Check sheet for the modelled part. Datum: model origin and axes. Units: mm. Coordinates: 2 decimals unless noted, no trailing zeros. Loops run counter-clockwise (first coordinate to the right, second up) from the corner with the lowest first, then second, coordinate; pieces in that order, holes last. Notation, with made-up numbers: M 20,84 L 77,84 A17 cw 77,93 Z; hole C 19,-40 d10. An arc over 180 degrees is marked long. Use CSV: the item, a comma, the result in double quotes. Start each with the question number.
(1) Scan lines: line 1 (Z direction, x = 9, y = 4.25); line 2 (Z direction, x = -8.5, y = 5.25); line 3 (Z direction, x = -76.5, y = 9.25). Record each from-to range of solid material in increasing order.
(2) Go/stop test with flat-tipped pins: pin 1 Ø6.5 at (y, z) = (4.5, -38) entering from -X; pin 2 Ø12 at (x, z) = (12.5, 74.5) entering from +Y; pin 3 Ø2 at (y, z) = (6, -51.5) entering from -X. Record where each tip stops, or that it passes through.
(3) Section check B-B on x = -17. Record the cut outline in (y, z), and give its area (3 significant figures).
(4) Section check C-C on z = 66. Record the cut outline in (x, y).
(5) Section check D-D on y = 2.5. Give the number of separate pieces and of enclosed holes in the cut face, and give its area (3 significant figures).
(6) Draft check along X on faces 1 (the flat face through (-74, 10, 62)), 2 (the flat face through (-89.5, 5, -39)), 3 (the cylindrical face through (-3.905, 6.338, -0.867)), 4 (the flat face through (89.5, 5, -47)). Enter one of: pulls with the +X half, pulls with the -X half, needs draft (parallel to the pull), parting line crosses it, or undercut.
(7) Section check A-A on x = -42.5. Record the cut outline in (y, z).
from build123d import *

# Parameters (mm, degrees)
SKETCH1_W               = 32.5
SKETCH1_H               = 40
SKETCH1_R               = 1.55
SKETCH1_W_2             = 40
SKETCH1_H_2             = 32.75
BOSS_EXTRUDE1_DEPTH     = 10
BOSS_EXTRUDE2_DEPTH     = 12.5
SKETCH3_R               = 4
CUT_EXTRUDE1_DEPTH      = 12.5
FILL_PATTERN1_OUTLINE_R = 4
FILL_PATTERN1_DEPTH     = 12.5
FILLET1_R               = 10
FILLET2_R               = 2


# Read off the part's stored shape, not the designer's step: Fill Pattern1
with BuildPart() as part:
    # Sketch1 → Boss-Extrude1 (new body)
    # profile 1 of 9: a face of its own
    with BuildSketch(Plane(origin=(0, 0, 0), x_dir=(1, 0, 0), z_dir=(0, 1, 0))):
        with BuildLine():
            Line((-35, 62.25), (-72, 62.25))
            ThreePointArc((-72, 62.25), (-77.125631329, 49.875631329), (-89.5, 44.75))
            Line((-89.5, 44.75), (-89.5, 35))
            Line((-89.5, 35), (-86.5, 35))
            Line((-86.5, 35), (-86.5, 20))
            Line((-86.5, 20), (-57, 20))
            Line((-57, 20), (-57, -20))
            Line((-57, -20), (-86.5, -20))
            Line((-86.5, -20), (-86.5, -35))
            Line((-86.5, -35), (-89.5, -35))
            Line((-89.5, -35), (-89.5, -62.25))
            Line((-89.5, -62.25), (-35, -62.25))
            Line((-35, -62.25), (-35, -59.25))
            Line((-35, -59.25), (-20, -59.25))
            Line((-20, -59.25), (-20, -29.5))
            Line((-20, -29.5), (20, -29.5))
            Line((20, -29.5), (20, -59.25))
            Line((20, -59.25), (35, -59.25))
            Line((35, -59.25), (35, -62.25))
            Line((35, -62.25), (89.5, -62.25))
            Line((89.5, -62.25), (89.5, -35))
            Line((89.5, -35), (86.5, -35))
            Line((86.5, -35), (86.5, -20))
            Line((86.5, -20), (57, -20))
            Line((57, -20), (57, 20))
            Line((57, 20), (86.5, 20))
            Line((86.5, 20), (86.5, 35))
            Line((86.5, 35), (89.5, 35))
            Line((89.5, 35), (89.5, 62.25))
            Line((89.5, 62.25), (35, 62.25))
            Line((35, 62.25), (35, 59.25))
            Line((35, 59.25), (20, 59.25))
            Line((20, 59.25), (20, 29.5))
            Line((20, 29.5), (-20, 29.5))
            Line((-20, 29.5), (-20, 59.25))
            Line((-20, 59.25), (-35, 59.25))
            Line((-35, 59.25), (-35, 62.25))
        make_face()
    # profile 2 of 9: a face of its own
    with BuildSketch(Plane(origin=(0, 0, 0), x_dir=(1, 0, 0), z_dir=(0, 1, 0))):
        Polygon((89.5, -20), (89.5, 20), (86.5, 20), (57, 20), (57, -20), (86.5, -20), align=None)
    # profile 3 of 9: a face of its own
    with BuildSketch(Plane(origin=(0, 0, 0), x_dir=(1, 0, 0), z_dir=(0, 1, 0))):
        with Locations((105.75, 0)):
            Rectangle(SKETCH1_W, SKETCH1_H)
        with Locations(Location((102, 0, 0), (0, 0, 270))):
            Circle(SKETCH1_R, mode=Mode.SUBTRACT)
    # profile 4 of 9: a face of its own
    with BuildSketch(Plane(origin=(0, 0, 0), x_dir=(1, 0, 0), z_dir=(0, 1, 0))):
        Polygon((-20, -29.5), (-20, -59.25), (-20, -62.25), (20, -62.25), (20, -59.25), (20, -29.5), align=None)
    # profile 5 of 9: a face of its own
    with BuildSketch(Plane(origin=(0, 0, 0), x_dir=(1, 0, 0), z_dir=(0, 1, 0))):
        with Locations((0, -78.625)):
            Rectangle(SKETCH1_W_2, SKETCH1_H_2)
        with Locations(Location((0, -74.75, 0), (0, 0, 270))):
            Circle(SKETCH1_R, mode=Mode.SUBTRACT)
    # profile 6 of 9: a face of its own
    with BuildSketch(Plane(origin=(0, 0, 0), x_dir=(1, 0, 0), z_dir=(0, 1, 0))):
        Polygon((-86.5, 20), (-89.5, 20), (-89.5, -20), (-86.5, -20), (-57, -20), (-57, 20), align=None)
    # profile 7 of 9: a face of its own
    with BuildSketch(Plane(origin=(0, 0, 0), x_dir=(1, 0, 0), z_dir=(0, 1, 0))):
        with Locations((-105.75, 0)):
            Rectangle(SKETCH1_W, SKETCH1_H)
        with Locations(Location((-102, 0, 0), (0, 0, 270))):
            Circle(SKETCH1_R, mode=Mode.SUBTRACT)
    # profile 8 of 9: a face of its own
    with BuildSketch(Plane(origin=(0, 0, 0), x_dir=(1, 0, 0), z_dir=(0, 1, 0))):
        Polygon((20, 62.25), (-20, 62.25), (-20, 59.25), (-20, 29.5), (20, 29.5), (20, 59.25), align=None)
    # profile 9 of 9: a face of its own
    with BuildSketch(Plane(origin=(0, 0, 0), x_dir=(1, 0, 0), z_dir=(0, 1, 0))):
        with Locations((0, 78.625)):
            Rectangle(SKETCH1_W_2, SKETCH1_H_2)
        with Locations(Location((0, 74.75, 0), (0, 0, 270))):
            Circle(SKETCH1_R, mode=Mode.SUBTRACT)
    extrude(amount=BOSS_EXTRUDE1_DEPTH)

    # Sketch2 → Boss-Extrude2 (add)
    with BuildSketch(Plane(origin=(0, 0, 0), x_dir=(1, 0, 0), z_dir=(0, 1, 0))):
        with BuildLine():
            Line((35, -60.85), (87.5, -60.85))
            Line((87.5, -60.85), (87.5, -35))
            Line((87.5, -35), (86.5, -35))
            Line((86.5, -35), (86.5, -20))
            Line((86.5, -20), (87.5, -20))
            Line((87.5, -20), (87.5, 20))
            Line((87.5, 20), (86.5, 20))
            Line((86.5, 20), (86.5, 35))
            Line((86.5, 35), (87.5, 35))
            Line((87.5, 35), (87.5, 60.85))
            Line((87.5, 60.85), (35, 60.85))
            Line((35, 60.85), (35, 59.25))
            Line((35, 59.25), (20, 59.25))
            Line((20, 59.25), (20, 60.85))
            Line((20, 60.85), (-20, 60.85))
            Line((-20, 60.85), (-20, 59.25))
            Line((-20, 59.25), (-35, 59.25))
            Line((-35, 59.25), (-35, 60.85))
            Line((-35, 60.85), (-72.056089888, 60.85))
            ThreePointArc((-72.056089888, 60.85), (-76.914326674, 50.09060746), (-87.5, 44.864661349))
            Line((-87.5, 44.864661349), (-87.5, 35))
            Line((-87.5, 35), (-86.5, 35))
            Line((-86.5, 35), (-86.5, 20))
            Line((-86.5, 20), (-87.5, 20))
            Line((-87.5, 20), (-87.5, -20))
            Line((-87.5, -20), (-86.5, -20))
            Line((-86.5, -20), (-86.5, -35))
            Line((-86.5, -35), (-87.5, -35))
            Line((-87.5, -35), (-87.5, -60.85))
            Line((-87.5, -60.85), (-35, -60.85))
            Line((-35, -60.85), (-35, -59.25))
            Line((-35, -59.25), (-20, -59.25))
            Line((-20, -59.25), (-20, -60.85))
            Line((-20, -60.85), (20, -60.85))
            Line((20, -60.85), (20, -59.25))
            Line((20, -59.25), (35, -59.25))
            Line((35, -59.25), (35, -60.85))
        make_face()
    extrude(amount=BOSS_EXTRUDE2_DEPTH)

    # Sketch3 → Cut-Extrude1 (cut)
    with BuildSketch(Plane(origin=(0, 12.5, 0), x_dir=(1, 0, 0), z_dir=(0, 1, 0))):
        with Locations(Location((0, 0, 0), (0, 0, 270))):
            Circle(SKETCH3_R)
    extrude(amount=-CUT_EXTRUDE1_DEPTH, mode=Mode.SUBTRACT)

    # Fill Pattern1 outline → Fill Pattern1 (cut)
    with BuildSketch(Plane(origin=(0, 0, 0), x_dir=(1, 0, 0), z_dir=(0, 1, 0))):
        with Locations((76.5, -44.167295593)):
            Circle(FILL_PATTERN1_OUTLINE_R)
        with Locations((34, 29.444863729)):
            Circle(FILL_PATTERN1_OUTLINE_R)
        with Locations((42.5, 44.167295593)):
            Circle(FILL_PATTERN1_OUTLINE_R)
        with Locations((8.5, -44.167295593)):
            Circle(FILL_PATTERN1_OUTLINE_R)
        with Locations((17, -29.444863729)):
            Circle(FILL_PATTERN1_OUTLINE_R)
        with Locations((25.5, -14.722431864)):
            Circle(FILL_PATTERN1_OUTLINE_R)
        with Locations((34, 0)):
            Circle(FILL_PATTERN1_OUTLINE_R)
        with Locations((42.5, 14.722431864)):
            Circle(FILL_PATTERN1_OUTLINE_R)
        with Locations((51, 29.444863729)):
            Circle(FILL_PATTERN1_OUTLINE_R)
        with Locations((-8.5, -44.167295593)):
            Circle(FILL_PATTERN1_OUTLINE_R)
        with Locations((25.5, 44.167295593)):
            Circle(FILL_PATTERN1_OUTLINE_R)
        with Locations((17, 29.444863729)):
            Circle(FILL_PATTERN1_OUTLINE_R)
        with Locations((8.5, 14.722431864)):
            Circle(FILL_PATTERN1_OUTLINE_R)
        with Locations((0, -29.444863729)):
            Circle(FILL_PATTERN1_OUTLINE_R)
        with Locations((8.5, -14.722431864)):
            Circle(FILL_PATTERN1_OUTLINE_R)
        with Locations((17, 0)):
            Circle(FILL_PATTERN1_OUTLINE_R)
        with Locations((25.5, 14.722431864)):
            Circle(FILL_PATTERN1_OUTLINE_R)
        with Locations((42.5, -44.167295593)):
            Circle(FILL_PATTERN1_OUTLINE_R)
        with Locations((51, -29.444863729)):
            Circle(FILL_PATTERN1_OUTLINE_R)
        with Locations((59.5, -14.722431864)):
            Circle(FILL_PATTERN1_OUTLINE_R)
        with Locations((68, 0)):
            Circle(FILL_PATTERN1_OUTLINE_R)
        with Locations((76.5, -14.722431864)):
            Circle(FILL_PATTERN1_OUTLINE_R)
        with Locations((68, -29.444863729)):
            Circle(FILL_PATTERN1_OUTLINE_R)
        with Locations((59.5, -44.167295593)):
            Circle(FILL_PATTERN1_OUTLINE_R)
        with Locations((76.5, 14.722431864)):
            Circle(FILL_PATTERN1_OUTLINE_R)
        with Locations((42.5, -14.722431864)):
            Circle(FILL_PATTERN1_OUTLINE_R)
        with Locations((34, -29.444863729)):
            Circle(FILL_PATTERN1_OUTLINE_R)
        with Locations((25.5, -44.167295593)):
            Circle(FILL_PATTERN1_OUTLINE_R)
        with Locations((59.5, 44.167295593)):
            Circle(FILL_PATTERN1_OUTLINE_R)
        with Locations((51, 0)):
            Circle(FILL_PATTERN1_OUTLINE_R)
        with Locations((59.5, 14.722431864)):
            Circle(FILL_PATTERN1_OUTLINE_R)
        with Locations((68, 29.444863729)):
            Circle(FILL_PATTERN1_OUTLINE_R)
        with Locations((76.5, 44.167295593)):
            Circle(FILL_PATTERN1_OUTLINE_R)
        with Locations((-76.5, -44.167295593)):
            Circle(FILL_PATTERN1_OUTLINE_R)
        with Locations((-68, -29.444863729)):
            Circle(FILL_PATTERN1_OUTLINE_R)
        with Locations((-59.5, -14.722431864)):
            Circle(FILL_PATTERN1_OUTLINE_R)
        with Locations((-51, 0)):
            Circle(FILL_PATTERN1_OUTLINE_R)
        with Locations((-59.5, -44.167295593)):
            Circle(FILL_PATTERN1_OUTLINE_R)
        with Locations((-25.5, 44.167295593)):
            Circle(FILL_PATTERN1_OUTLINE_R)
        with Locations((-34, 29.444863729)):
            Circle(FILL_PATTERN1_OUTLINE_R)
        with Locations((-42.5, 14.722431864)):
            Circle(FILL_PATTERN1_OUTLINE_R)
        with Locations((-76.5, -14.722431864)):
            Circle(FILL_PATTERN1_OUTLINE_R)
        with Locations((-59.5, 44.167295593)):
            Circle(FILL_PATTERN1_OUTLINE_R)
        with Locations((-68, 29.444863729)):
            Circle(FILL_PATTERN1_OUTLINE_R)
        with Locations((-76.5, 14.722431864)):
            Circle(FILL_PATTERN1_OUTLINE_R)
        with Locations((-68, 0)):
            Circle(FILL_PATTERN1_OUTLINE_R)
        with Locations((-59.5, 14.722431864)):
            Circle(FILL_PATTERN1_OUTLINE_R)
        with Locations((-51, 29.444863729)):
            Circle(FILL_PATTERN1_OUTLINE_R)
        with Locations((-42.5, 44.167295593)):
            Circle(FILL_PATTERN1_OUTLINE_R)
        with Locations((-25.5, -14.722431864)):
            Circle(FILL_PATTERN1_OUTLINE_R)
        with Locations((-17, 0)):
            Circle(FILL_PATTERN1_OUTLINE_R)
        with Locations((-8.5, 14.722431864)):
            Circle(FILL_PATTERN1_OUTLINE_R)
        with Locations((0, 29.444863729)):
            Circle(FILL_PATTERN1_OUTLINE_R)
        with Locations((-8.5, -14.722431864)):
            Circle(FILL_PATTERN1_OUTLINE_R)
        with Locations((-17, -29.444863729)):
            Circle(FILL_PATTERN1_OUTLINE_R)
        with Locations((-25.5, -44.167295593)):
            Circle(FILL_PATTERN1_OUTLINE_R)
        with Locations((8.5, 44.167295593)):
            Circle(FILL_PATTERN1_OUTLINE_R)
        with Locations((-51, -29.444863729)):
            Circle(FILL_PATTERN1_OUTLINE_R)
        with Locations((-42.5, -14.722431864)):
            Circle(FILL_PATTERN1_OUTLINE_R)
        with Locations((-34, 0)):
            Circle(FILL_PATTERN1_OUTLINE_R)
        with Locations((-25.5, 14.722431864)):
            Circle(FILL_PATTERN1_OUTLINE_R)
        with Locations((-17, 29.444863729)):
            Circle(FILL_PATTERN1_OUTLINE_R)
        with Locations((-8.5, 44.167295593)):
            Circle(FILL_PATTERN1_OUTLINE_R)
        with Locations((-42.5, -44.167295593)):
            Circle(FILL_PATTERN1_OUTLINE_R)
        with Locations((-34, -29.444863729)):
            Circle(FILL_PATTERN1_OUTLINE_R)
    extrude(amount=FILL_PATTERN1_DEPTH, mode=Mode.SUBTRACT)

    # Fillet1
    fillet1_edges = [part.edges().sort_by_distance(p)[0] for p in [
        (-122, 5, 20),
        (-122, 5, -20),
        (-20, 5, -95),
        (20, 5, -95),
        (122, 5, -20),
        (122, 5, 20),
        (20, 5, 95),
        (-20, 5, 95),
    ]]
    fillet(fillet1_edges, radius=FILLET1_R)

    # Fillet2
    fillet2_edges = [part.edges().sort_by_distance(p)[0] for p in [
        (-89.5, 5, 62.25),
        (-89.5, 5, -44.75),
        (-72, 5, -62.25),
        (89.5, 5, -62.25),
    ]]
    fillet(fillet2_edges, radius=FILLET2_R)


solid = part.part
Outcome:
1,line 1,"z = -95 to -48.14, -40.2 to -18.69, -10.75 to 10.75, 18.69 to 40.2, 48.14 to 95"
1,line 2,"z = -95 to -48.17, -40.17 to -18.72, -10.72 to 10.72, 18.72 to 40.17, 48.17 to 95"
1,line 3,"z = -50.53 to -18.72, -10.72 to 10.72, 18.72 to 40.17, 48.17 to 62.25"
2,pin 1,"stops at x = -89.5"
2,pin 2,"stops at y = 10"
2,pin 3,"stops at x = -76.53"
3,outline,"M 0,-92.14 L 10,-92.14 L 10,-60.85 L 12.5,-60.85 L 12.5,-33.44 L 0,-33.44 Z; M 0,-25.44 L 12.5,-25.44 L 12.5,-4 L 0,-4 Z; M 0,4 L 12.5,4 L 12.5,25.44 L 0,25.44 Z; M 0,33.44 L 12.5,33.44 L 12.5,60.85 L 10,60.85 L 10,92.14 L 0,92.14 Z"
3,area,"1,850 mm²"
4,outline,"M -20,0 L 20,0 L 20,10 L -20,10 Z"
5,separate pieces,"1"
5,enclosed holes,"70"
5,area,"23,400 mm²"
6,face 1,"needs draft"
6,face 2,"pulls with the -X half"
6,face 3,"undercut"
6,face 4,"pulls with the +X half"
7,outline,"M 0,-62.25 L 10,-62.25 L 10,-60.85 L 12.5,-60.85 L 12.5,-48.17 L 0,-48.17 Z; M 0,-40.17 L 12.5,-40.17 L 12.5,-18.72 L 0,-18.72 Z; M 0,-10.72 L 12.5,-10.72 L 12.5,10.72 L 0,10.72 Z; M 0,18.72 L 12.5,18.72 L 12.5,40.17 L 0,40.17 Z; M 0,48.17 L 12.5,48.17 L 12.5,60.85 L 10,60.85 L 10,62.25 L 0,62.25 Z"
